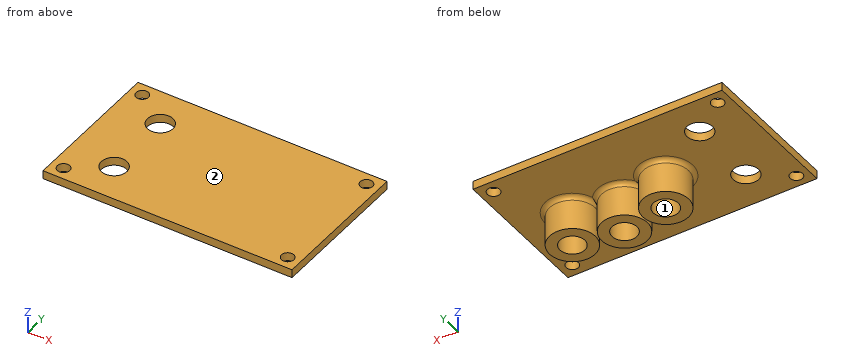
```python
from build123d import *

# Parameters (mm, degrees)
SKETCH1_W           = 60
SKETCH1_H           = 35
SKETCH1_R           = 1.5
BOSS_EXTRUDE1_DEPTH = 2
SKETCH2_R           = 5.5
BOSS_EXTRUDE2_DEPTH = 8.2
SKETCH5_R           = 3
CUT_EXTRUDE2_DEPTH  = 8.2
SKETCH6_R           = 3.075
CUT_EXTRUDE3_DEPTH  = 8.2
FILLET4_R           = 1


with BuildPart() as part:
    # Sketch1 → Boss-Extrude1 (new body)
    with BuildSketch(Plane.XY):
        with Locations((30, 17.5)):
            Rectangle(SKETCH1_W, SKETCH1_H)
        with Locations((57, 32)):
            Circle(SKETCH1_R, mode=Mode.SUBTRACT)
        with Locations((57, 3)):
            Circle(SKETCH1_R, mode=Mode.SUBTRACT)
        with Locations((3, 3)):
            Circle(SKETCH1_R, mode=Mode.SUBTRACT)
        with Locations((3, 32)):
            Circle(SKETCH1_R, mode=Mode.SUBTRACT)
    extrude(amount=BOSS_EXTRUDE1_DEPTH)

    # Sketch2 → Boss-Extrude2 (add)
    with BuildSketch(Plane(origin=(0, 0, 0), x_dir=(-1, 0, 0), z_dir=(0, 0, -1))):
        with Locations((-36.25, 15.5)):
            Circle(SKETCH2_R)
        with Locations((-25, 17.5)):
            Circle(SKETCH2_R)
        with Locations((-47.5, 17.5)):
            Circle(SKETCH2_R)
    extrude(amount=BOSS_EXTRUDE2_DEPTH)

    # Sketch5 → Cut-Extrude2 (cut)
    with BuildSketch(Plane(origin=(0, 0, -8.2), x_dir=(-1, 0, 0), z_dir=(0, 0, -1))):
        with Locations((-47.5, 17.5)):
            Circle(SKETCH5_R)
        with Locations((-36.25, 15.5)):
            Circle(SKETCH5_R)
        with Locations((-25, 17.5)):
            Circle(SKETCH5_R)
    extrude(amount=-CUT_EXTRUDE2_DEPTH, mode=Mode.SUBTRACT)

    # Sketch6 → Cut-Extrude3 (cut)
    with BuildSketch(Plane(origin=(0, 0, 0), x_dir=(-1, 0, 0), z_dir=(0, 0, -1))):
        with Locations((-11.25, 26)):
            Circle(SKETCH6_R)
        with Locations((-11.25, 9)):
            Circle(SKETCH6_R)
    extrude(amount=-CUT_EXTRUDE3_DEPTH, mode=Mode.SUBTRACT)

    # Fillet4
    # the kernel refuses this fillet: 1 mm, written as the material it adds along each edge
    with BuildSketch(Plane(origin=(36.25, 15.5, 0), x_dir=(-1, 0, 0), z_dir=(0, -1, 0))) as fillet4_piece_1:
        with BuildLine():
            CenterArc((5.5 + FILLET4_R, FILLET4_R), FILLET4_R, 180, 90)
            Line((5.5, FILLET4_R), (5.5, 0))
            Line((5.5, 0), (5.5 + FILLET4_R, 0))
        make_face()
    revolve(axis=Axis((36.25, 15.5, 0), (0, 0, -1)))
    with BuildSketch(Plane(origin=(25, 17.5, 0), x_dir=(-1, 0, 0), z_dir=(0, -1, 0))) as fillet4_piece_2:
        with BuildLine():
            CenterArc((5.5 + FILLET4_R, FILLET4_R), FILLET4_R, 180, 90)
            Line((5.5, FILLET4_R), (5.5, 0))
            Line((5.5, 0), (5.5 + FILLET4_R, 0))
        make_face()
    revolve(axis=Axis((25, 17.5, 0), (0, 0, -1)))
    with BuildSketch(Plane(origin=(47.5, 17.5, 0), x_dir=(-1, 0, 0), z_dir=(0, -1, 0))) as fillet4_piece_3:
        with BuildLine():
            CenterArc((5.5 + FILLET4_R, FILLET4_R), FILLET4_R, 180, 90)
            Line((5.5, FILLET4_R), (5.5, 0))
            Line((5.5, 0), (5.5 + FILLET4_R, 0))
        make_face()
    revolve(axis=Axis((47.5, 17.5, 0), (0, 0, -1)))


solid = part.part
```
CAD build for the part. Positions are in the model's coordinates, mm. Face numbers are marked on the shaded views. Give positions to 0.01 mm unless a question says otherwise; leave off trailing zeros. Write each loop counter-clockwise with the first axis right and the second up, starting at its lowest first coordinate (ties: lowest second). Pieces come first, ordered by that corner, then holes. Notation, with made-up numbers: (64.25, 54) -> (91.25, 54) arc R23 ccw to (91.25, 76) -> close; hole circle Ø4 at (61.5, 49.25). An arc over 180 degrees is marked (long way). Write each question's results on one line, items separated by ' | '.
1. Cut at A-A, the plane x = 11.25. Write the cut outline in (y, z) (3 decimals).
Geometry check:
outline: (0, 0) -> (5.925, 0) -> (5.925, 2) -> (0, 2) -> close; (12.075, 0) -> (22.925, 0) -> (22.925, 2) -> (12.075, 2) -> close; (29.075, 0) -> (35, 0) -> (35, 2) -> (29.075, 2) -> close
2. Wall check: probe 1 along Y at (x, z) = (3, 1.25); probe 2 along Y at (x, z) = (25, -4.75); probe 3 along X at (y, z) = (2, 1.5). Give the ranges that are in metal, low to high. Write a range as [from, to].
Geometry check:
probe 1: [0, 1.5], [4.5, 30.5], [33.5, 35] | probe 2: [12, 14.5], [20.5, 23] | probe 3: [0, 1.88], [4.12, 55.88], [58.12, 60]
3. Two-plate mould, pull along X, no slides. Class the marked faces 1 and 2: pulls with the +X half, pulls with the -X half, needs draft (parallel to the pull), parting line crosses it, or undercut.
Geometry check:
face 1: undercut | face 2: needs draft
4. Cut at B-B, the plane z = -5. Write the cut outline in (x, y).
Geometry check:
outline: circle Ø11 at (25, 17.5); circle Ø11 at (36.25, 15.5); circle Ø11 at (47.5, 17.5); hole circle Ø6 at (25, 17.5); hole circle Ø6 at (36.25, 15.5); hole circle Ø6 at (47.5, 17.5)
5. Drop flat-ended pins along their axis: P1, Ø5, axis at x = 25, y = 17.5, coming from the -Z side; P2, Ø3, axis at y = 29, z = 0.5, coming from the -X side; P3, Ø2, axis at y = 9.5, z = -3.5, coming from the -X side; P4, Ø6, axis at y = 11.5, z = -5, coming from the +X side. Give the stop position or say it passes through.
Geometry check:
P1: z = 0 | P2: x = 0 | P3: x = 33.96 | P4: x = 52.11
6. Cut at D-D, the plane x = 25. Write the cut outline in (y, z), then the cut area to 3 significant figures.
Geometry check:
outline: (0, 0) -> (11, 0) arc R1 cw to (12, -1) -> (12, -8.2) -> (14.5, -8.2) -> (14.5, 0) -> (20.5, 0) -> (20.5, -8.2) -> (23, -8.2) -> (23, -1) arc R1 cw to (24, 0) -> (35, 0) -> (35, 2) -> (0, 2) -> close | area: 111 mm²
7. Cut at C-C, the plane y = 32. Write the cut outline in (x, z).
Geometry check:
outline: (0, 0) -> (1.5, 0) -> (1.5, 2) -> (0, 2) -> close; (4.5, 0) -> (55.5, 0) -> (55.5, 2) -> (4.5, 2) -> close; (58.5, 0) -> (60, 0) -> (60, 2) -> (58.5, 2) -> close
